Part model, mm, in its own coordinate system. Give positions to 0.01 mm unless a question says otherwise; leave off trailing zeros. Order: outer loops, then holes, each group sorted by start corner. A loop starts at its lowest first (then second) coordinate and runs counter-clockwise, first axis right, second up. Notation, with made-up numbers: M 23,-27 L 56,-27 A29 ccw 56,1 Z; hole C 18.5,79 d7. An arc over 180 degrees is marked long. Return JSON: item names as keys, results as strings.
Autodesk Inventor part; units mm, degrees
ref_plane "YZ Plane" through (0, 0, 0) normal (1, 0, 0) x (0, 1, 0)
ref_plane "XZ Plane" through (0, 0, 0) normal (0, 1, 0) x (-1, 0, 0)
ref_plane "XY Plane" through (0, 0, 0) normal (0, 0, 1) x (1, 0, 0)
sketch "Skizze2" plane through (0, 0, 0) normal (0, 0, 1) x (1, 0, 0)
  circle A0 centre (0, 0) radius 5
  dimension "d0" = 10
extrude "Extrusion1" add sketch "Skizze2" along normal mid plane 505
sketch "Skizze3" plane through (0, 0, -252.5) normal (0, 0, -1) x (-1, 0, 0)
  point P0 (0, 0)
  point P1 (0, 0)
hole "Bohrung1" at (0, 0, -252.5) direction (0, 0, 1) diameter 4.917 depth 12 tip angle 118
chamfer "Fasen1" distance 0.5 angle 45 3 edges at (0, -2.4585, -252.5) (-5, 0, -252.5) (-5, 0, 252.5)
equation "\"d0\" = Durchmesser_fuehrungsstab"
equation "\"d1\" = Hoehe_Magazin + Fuehrung_Bodenplatte"
equation "\"d4\" = Tiefe_Bohrung"
equation "\"d10\" = Fase"
equation "\"Durchmesser_fuehrungsstab\" = 10"
equation "\"Hoehe_Magazin\" = 500"
equation "\"Tiefe_Bohrung\" = 10"
equation "\"Fuehrung_Bodenplatte\" = 5"
equation "\"Fase\" = 0.5"
properties part number "TS_Magazin_Fuehrungselement_int"
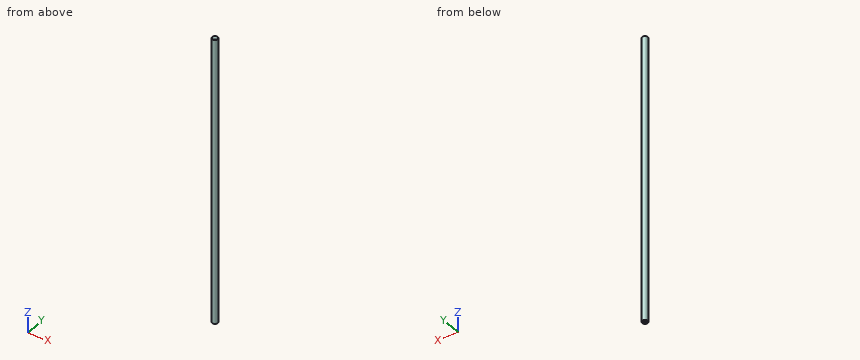
Q1. Probe line 1 along Y through (x, z) = (0, -243.5); line 2 along Z through (x, y) = (-3.75, 3.25); line 3 along Y through (x, z) = (4, -38.5). List the from-to ranges inside material, lowest first.
Established:
{"line 1": "y = -5 to -2.46, 2.46 to 5", "line 2": "z = -252.04 to 252.04", "line 3": "y = -3 to 3"}
Q2. Pin check, flat tips, straight feed: pin 1 (2 mm diameter, centred on y = -3.5, z = 69, fed in from +X); pin 2 (3 mm diameter, centred on y = 2, z = 120, fed in from -X). Stop position of each tip, or through.
Established:
{"pin 1": "stops at x = 4.33", "pin 2": "stops at x = -4.97"}
Q3. Band-saw the part on A-A (z = -79). Give the cut face in (x, y).
Established:
{"outline": "C 0,0 d10"}
